from build123d import *

# Parameters (mm, degrees)
SKETCH1_W          = 203.2
SKETCH1_H          = 50.8
BASE_FLANGE1_DEPTH = 1.5875
EDGE_FLANGE3_DEPTH = 203.2
SKETCH15_R         = 3.175
CUT_EXTRUDE1_DEPTH = 1.5875


# Sheet-metal steps are written as plain solids
with BuildPart() as part:
    # Sketch1 → Base-Flange1 (new body)
    with BuildSketch(Plane(origin=(0, 0, 0), x_dir=(1, 0, 0), z_dir=(0, 1, 0))):
        with Locations((12.472748517, 25.4)):
            Rectangle(SKETCH1_W, SKETCH1_H)
    extrude(amount=-BASE_FLANGE1_DEPTH)

    # Edge-Flange3 section (across the edge) → Edge-Flange3 (add)
    with BuildSketch(Plane(origin=(-89.127251483, 0, 0.7366), x_dir=(0, 0, -1), z_dir=(1, 0, 0))):
        with BuildLine():
            Line((-1.5875, 0.7366), (-1.5875, 49.2125))
            Line((-1.5875, 49.2125), (0, 49.2125))
            Line((0, 49.2125), (0, 0.7366))
            ThreePointArc((0, 0.7366), (0.215745145, 0.215745145), (0.7366, 0))
            Line((0.7366, 0), (0.7366, -1.5875))
            ThreePointArc((0.7366, -1.5875), (-0.90678687, -0.90678687), (-1.5875, 0.7366))
        make_face()
    extrude(amount=EDGE_FLANGE3_DEPTH)

    # Sketch15 → Cut-Extrude1 (cut)
    with BuildSketch(Plane(origin=(0, 0, 0), x_dir=(1, 0, 0), z_dir=(0, 1, 0))):
        with Locations(Location((-51.027251483, 38.1, 0), (0, 0, 270))):
            Circle(SKETCH15_R)
        with Locations(Location((75.972748517, 38.1, 0), (0, 0, 270))):
            Circle(SKETCH15_R)
        with Locations(Location((-51.027251483, 12.7, 0), (0, 0, 270))):
            Circle(SKETCH15_R)
        with Locations(Location((75.972748517, 12.7, 0), (0, 0, 270))):
            Circle(SKETCH15_R)
    extrude(amount=-CUT_EXTRUDE1_DEPTH, mode=Mode.SUBTRACT)


solid = part.part
Source: CAD feature listing. Evaluate the final solid. Frame: model axes, mm. A direction names the side the tool comes from. Round coordinates to 2 decimals unless told otherwise and drop trailing zeros. Write each loop counter-clockwise with the first axis right and the second up, starting at its lowest first coordinate (ties: lowest second). Pieces come first, ordered by that corner, then holes. Notation, with made-up numbers: M 86.5,51.25 L 102.5,51.25 A10 ccw 102.5,58.25 Z; hole C -17,23.5 d9. An arc over 180 degrees is marked long. One line per item, written item: value. Start each with the question number.
Item 1: Mould query, pull axis X, two halves, no side actions, for faces 1 (the flat face through (11, 0, -26)), 2 (the cylindrical face through (-47.88, -0.78, -13.11)), 3 (the cylindrical face through (72.873, -0.783, -38.788)), 4 (the flat face through (-89.127, -1, -13)). Classes: pulls with the +X half, pulls with the -X half, needs draft (parallel to the pull), parting line crosses it, or undercut.
Item 2: Pin query (flat end, axial travel): pin 1 (14.5 mm diameter, centred on x = 3, y = 18.5, fed in from -Z); pin 2 (7.5 mm diameter, centred on x = 75.97, z = -12.7, fed in from +Y). Return the tip coordinate at first contact, or that it passes through.
Item 3: Set-up query: faces 5 (the flat face through (11, -1.588, -26)), 6 (the flat face through (11, 25, 0.737)). Return all of +Z, -Z, +X, -X, +Y, -Y with unobstructed straight access to the full face (end or side cutting, diameter ignored); none if empty.
Item 4: Section query C-C (z = -28.5). Return the cut outline in (x, y).
Item 5: Section query B-B (x = 37.5). Return the cut outline in (y, z), plus the area to 3 significant figures.
Item 6: Section query D-D (z = -12.5). Return the cut outline in (x, y).
Item 7: Ray query, L1, parallel to X at y = -0.9, z = -12.7; L2, parallel to Y at x = -59, z = -16; L3, parallel to Z at x = 33, y = 44. Return the intervals inside material, ascending. Write a range as from..to.
Item 8: Section query A-A (z = -38.1). Return the cut outline in (x, y).
Result set:
1. face 1: needs draft
1. face 2: undercut
1. face 3: undercut
1. face 4: pulls with the -X half
2. pin 1: stops at z = 0.74
2. pin 2: stops at y = 0
3. face 5: +Z, -Z, +X, -X, -Y
3. face 6: -Z, +X, -X, +Y
4. outline: M -89.13,-1.59 L 114.07,-1.59 L 114.07,0 L -89.13,0 Z
5. outline: M -1.59,-50.8 L 0,-50.8 L 0,0 A0.74 cw 0.74,0.74 L 49.21,0.74 L 49.21,2.32 L 0.74,2.32 A2.32 ccw -1.59,0 Z
5. area: 161 mm²
6. outline: M -89.13,-1.59 L -54.2,-1.59 L -54.2,0 L -89.13,0 Z; M -47.86,-1.59 L 72.8,-1.59 L 72.8,0 L -47.86,0 Z; M 79.14,-1.59 L 114.07,-1.59 L 114.07,0 L 79.14,0 Z
7. L1: x = -89.13..-54.2, -47.85..72.8, 79.15..114.07
7. L2: y = -1.59..0
7. L3: z = 0.74..2.32
8. outline: M -89.13,-1.59 L -54.2,-1.59 L -54.2,0 L -89.13,0 Z; M -47.85,-1.59 L 72.8,-1.59 L 72.8,0 L -47.85,0 Z; M 79.15,-1.59 L 114.07,-1.59 L 114.07,0 L 79.15,0 Z
